Read the model definition and answer for the solid it produces. Units are mm, in the model's axes. Face numbers are marked on the shaded views. A direction names the side the tool comes from. Round coordinates to 2 decimals unless told otherwise and drop trailing zeros. Loops run counter-clockwise (first coordinate to the right, second up) from the corner with the lowest first, then second, coordinate; pieces in that order, holes last. Notation, with made-up numbers: M 3.25,84 L 60.25,84 A31 cw 60.25,111 Z; hole C 52.5,54.25 d5. An arc over 180 degrees is marked long. Write each question's results on one line, items separated by ' | '.
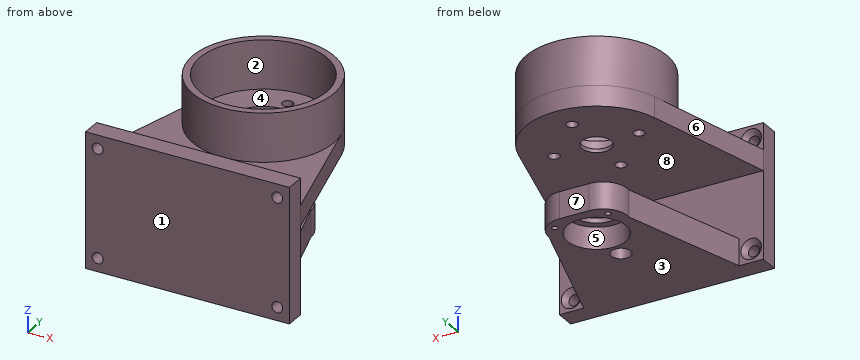
```python
from build123d import *

# Parameters (mm, degrees)
SCHIZZO1_R                   = 12.1
ESTRUSIONE_ESTRUSIONE1_DEPTH = 11
ESTRUSIONE_ESTRUSIONE2_START = -2
SCHIZZO2_R                   = 12.1
SCHIZZO2_R_2                 = 9
ESTRUSIONE_ESTRUSIONE2_DEPTH = 2
SCHIZZO3_R                   = 2.25
TAGLIO_ESTRUSIONE1_DEPTH     = 77.182412669
SMUSSO1_SIZE                 = 2
SCHIZZO4_R                   = 1.25
TAGLIO_ESTRUSIONE2_DEPTH     = 70.679623994
SCHIZZO5_W                   = 84
SCHIZZO5_H                   = 8
ESTRUSIONE_ESTRUSIONE3_DEPTH = 25
SCHIZZO6_R                   = 2.25
SCHIZZO6_R_2                 = 6
ESTRUSIONE_ESTRUSIONE4_DEPTH = 1.5
SCHIZZO7_R                   = 2.25
SCHIZZO7_R_2                 = 13.1
ESTRUSIONE_ESTRUSIONE5_DEPTH = 7
SCHIZZO8_R                   = 29
SCHIZZO8_R_2                 = 26.1
ESTRUSIONE_ESTRUSIONE6_DEPTH = 20
TAGLIO_ESTRUSIONE4_REACH     = 96.311
SCHIZZO9_R                   = 4
SCHIZZO10_W                  = 84
SCHIZZO10_H                  = 8
ESTRUSIONE_ESTRUSIONE7_DEPTH = 11
SCHIZZO11_R                  = 2.25
TAGLIO_ESTRUSIONE5_DEPTH     = 108.816974545
SMUSSO2_SIZE                 = 2


with BuildPart() as part:
    # Schizzo1 → Estrusione-Estrusione1 (new body)
    with BuildSketch(Plane.XY):
        with BuildLine():
            Line((-6.171311325, 16.1), (6.171311325, 16.1))
            ThreePointArc((6.171311325, 16.1), (13.242379137, 13.171067812), (16.171311325, 6.1))
            Line((16.171311325, 6.1), (32, -46.5))
            Line((32, -46.5), (42, -46.5))
            Line((42, -46.5), (42, -54.5))
            Line((42, -54.5), (17, -54.5))
            Line((17, -54.5), (-17, -54.5))
            Line((-17, -54.5), (-42, -54.5))
            Line((-42, -54.5), (-42, -46.5))
            Line((-42, -46.5), (-32, -46.5))
            Line((-32, -46.5), (-16.1, 4.907883736))
            ThreePointArc((-16.1, 4.907883736), (-13.651991863, 12.73622021), (-6.171311325, 16.1))
        make_face()
        Circle(SCHIZZO1_R, mode=Mode.SUBTRACT)
    extrude(amount=ESTRUSIONE_ESTRUSIONE1_DEPTH)

    # Schizzo2 → Estrusione-Estrusione2 (add)
    with BuildSketch(Plane.XY.offset(11).offset(ESTRUSIONE_ESTRUSIONE2_START)):
        Circle(SCHIZZO2_R)
        Circle(SCHIZZO2_R_2, mode=Mode.SUBTRACT)
    extrude(amount=ESTRUSIONE_ESTRUSIONE2_DEPTH)

    # Schizzo3 → Taglio-Estrusione1 (cut, through all)
    with BuildSketch(Plane(origin=(0, -46.5, 0), x_dir=(1, 0, 0), z_dir=(0, 1, 0))):
        with Locations(Location((37, -5.5, 0), (0, 0, 270))):
            Circle(SCHIZZO3_R)
        with Locations(Location((-37, -5.5, 0), (0, 0, 270))):
            Circle(SCHIZZO3_R)
    extrude(amount=-TAGLIO_ESTRUSIONE1_DEPTH, mode=Mode.SUBTRACT)

    # Smusso1
    smusso1_edges = [part.edges().sort_by_distance(p)[0] for p in [
        (37, -46.5, 3.25),
        (-37, -46.5, 3.25),
    ]]
    chamfer(smusso1_edges, length=SMUSSO1_SIZE)

    # Schizzo4 → Taglio-Estrusione2 (cut, through all)
    with BuildSketch(Plane(origin=(0, 0, 0), x_dir=(-1, 0, 0), z_dir=(0, 0, -1))):
        with Locations((-10.910719744, 10.851964601)):
            Circle(SCHIZZO4_R)
        with Locations((10.944459062, 10.817992606)):
            Circle(SCHIZZO4_R)
        with Locations((0, -15.38859776)):
            Circle(SCHIZZO4_R)
    extrude(amount=-TAGLIO_ESTRUSIONE2_DEPTH, mode=Mode.SUBTRACT)

    # Schizzo5 → Estrusione-Estrusione3 (add)
    with BuildSketch(Plane.XY.offset(11)):
        with Locations((0, -50.5)):
            Rectangle(SCHIZZO5_W, SCHIZZO5_H)
    extrude(amount=ESTRUSIONE_ESTRUSIONE3_DEPTH)

    # Schizzo6 → Estrusione-Estrusione4 (add)
    with BuildSketch(Plane.XY.offset(36)):
        with BuildLine():
            Line((-28.073726485, 7.270892739), (-42, -46.5))
            Line((-42, -46.5), (-42, -54.5))
            Line((-42, -54.5), (42, -54.5))
            Line((42, -54.5), (42, -46.5))
            Line((42, -46.5), (28.073726485, 7.270892739))
            ThreePointArc((28.073726485, 7.270892739), (0, 29), (-28.073726485, 7.270892739))
        make_face()
        with Locations((17.5, 0)):
            Circle(SCHIZZO6_R, mode=Mode.SUBTRACT)
        with Locations((0, -17.5)):
            Circle(SCHIZZO6_R, mode=Mode.SUBTRACT)
        with Locations((-17.5, 0)):
            Circle(SCHIZZO6_R, mode=Mode.SUBTRACT)
        with Locations((0, 17.5)):
            Circle(SCHIZZO6_R, mode=Mode.SUBTRACT)
        Circle(SCHIZZO6_R_2, mode=Mode.SUBTRACT)
    extrude(amount=ESTRUSIONE_ESTRUSIONE4_DEPTH)

    # Schizzo7 → Estrusione-Estrusione5 (add)
    with BuildSketch(Plane.XY.offset(37.5)):
        with BuildLine():
            Line((42, -46.5), (28.073726485, 7.270892739))
            ThreePointArc((28.073726485, 7.270892739), (0, 29), (-28.073726485, 7.270892739))
            Line((-28.073726485, 7.270892739), (-42, -46.5))
            Line((-42, -46.5), (-42, -54.5))
            Line((-42, -54.5), (42, -54.5))
            Line((42, -54.5), (42, -46.5))
        make_face()
        with Locations((0, -17.5)):
            Circle(SCHIZZO7_R, mode=Mode.SUBTRACT)
        with Locations((17.5, 0)):
            Circle(SCHIZZO7_R, mode=Mode.SUBTRACT)
        with Locations((0, 17.5)):
            Circle(SCHIZZO7_R, mode=Mode.SUBTRACT)
        with Locations((-17.5, 0)):
            Circle(SCHIZZO7_R, mode=Mode.SUBTRACT)
        Circle(SCHIZZO7_R_2, mode=Mode.SUBTRACT)
    extrude(amount=ESTRUSIONE_ESTRUSIONE5_DEPTH)

    # Schizzo8 → Estrusione-Estrusione6 (add)
    with BuildSketch(Plane.XY.offset(44.5)):
        with Locations(Location((0, 0, 0), (0, 0, 165.479851844))):
            Circle(SCHIZZO8_R)
        Circle(SCHIZZO8_R_2, mode=Mode.SUBTRACT)
    extrude(amount=ESTRUSIONE_ESTRUSIONE6_DEPTH)

    # Schizzo9 → Taglio-Estrusione4 (cut, up to next)
    with BuildSketch(Plane(origin=(0, 0, 0), x_dir=(-1, 0, 0), z_dir=(0, 0, -1)), mode=Mode.PRIVATE) as taglio_estrusione4_sk1:
        with Locations((0, -17.5)):
            Circle(SCHIZZO9_R)
    taglio_estrusione4_tool1 = extrude(taglio_estrusione4_sk1.sketch, amount=-TAGLIO_ESTRUSIONE4_REACH, mode=Mode.PRIVATE) & part.part
    add(taglio_estrusione4_tool1.solids().sort_by_distance((0, -17.5, 0))[0], mode=Mode.SUBTRACT)

    # Schizzo10 → Estrusione-Estrusione7 (add)
    with BuildSketch(Plane.XY.offset(44.5)):
        with Locations((0, -50.5)):
            Rectangle(SCHIZZO10_W, SCHIZZO10_H)
    extrude(amount=ESTRUSIONE_ESTRUSIONE7_DEPTH)

    # Schizzo11 → Taglio-Estrusione5 (cut, through all)
    with BuildSketch(Plane(origin=(0, -46.5, 0), x_dir=(1, 0, 0), z_dir=(0, 1, 0))):
        with Locations(Location((-37, -50, 0), (0, 0, 270))):
            Circle(SCHIZZO11_R)
        with Locations(Location((37, -50, 0), (0, 0, 270))):
            Circle(SCHIZZO11_R)
    extrude(amount=-TAGLIO_ESTRUSIONE5_DEPTH, mode=Mode.SUBTRACT)

    # Smusso2
    smusso2_edges = [part.edges().sort_by_distance(p)[0] for p in [
        (-37, -46.5, 47.75),
        (37, -46.5, 47.75),
    ]]
    chamfer(smusso2_edges, length=SMUSSO2_SIZE)


solid = part.part
```
1. Find section C-C, the plane x = 17.5. Give the vertices of the cut face in (y, z), then the cut area to 3 significant figures.
Completed:
outline: M -54.5,0 L 1.68,0 L 1.68,11 L -46.5,11 L -46.5,36 L -2.25,36 L -2.25,44.5 L -19.36,44.5 L -19.36,64.5 L -23.12,64.5 L -23.12,44.5 L -46.5,44.5 L -46.5,55.5 L -54.5,55.5 Z; M 2.25,36 L 23.12,36 L 23.12,64.5 L 19.36,64.5 L 19.36,44.5 L 2.25,44.5 Z | area: 1,680 mm2
2. Given P1, Ø6, axis at x = -11.5, z = 20.5, coming from the +Y side; P2, Ø22, axis at x = 0, y = 0, coming from the +Z side; P3, Ø5.5, axis at x = 1, z = 4, coming from the +Y side, each flat-ended and moving along its own axis, determine where each tip first touches the part or whether it passes through.
Completed:
P1: stops at y = -46.5 | P2: stops at z = 37.5 | P3: stops at y = 16.1
3. Find section A-A, the plane z = 5.5. Give the vertices of the cut face in (x, y).
Completed:
outline: M -42,-54.5 L -39.25,-54.5 L -39.25,-48.5 L -41.25,-46.5 L -42,-46.5 Z; M -34.75,-54.5 L 34.75,-54.5 L 34.75,-48.5 L 32.75,-46.5 L 32,-46.5 L 16.17,6.1 A10 ccw 6.17,16.1 L -6.17,16.1 A10 ccw -16.1,4.91 L -32,-46.5 L -32.75,-46.5 L -34.75,-48.5 Z; M 39.25,-54.5 L 42,-54.5 L 42,-46.5 L 41.25,-46.5 L 39.25,-48.5 Z; hole C -10.94,10.82 d2.5; hole C 0,0 d24.2; hole C 0,-17.5 d8; hole C 10.91,10.85 d2.5
4. Find section D-D, the plane x = -37. Give the vertices of the cut face in (y, z), then the cut area to 3 significant figures.
Completed:
outline: M -54.5,0 L -46.5,0 L -46.5,1.25 L -48.5,3.25 L -54.5,3.25 Z; M -54.5,7.75 L -48.5,7.75 L -46.5,9.75 L -46.5,36 L -27.19,36 L -27.19,44.5 L -46.5,44.5 L -46.5,45.75 L -48.5,47.75 L -54.5,47.75 Z; M -54.5,52.25 L -48.5,52.25 L -46.5,54.25 L -46.5,55.5 L -54.5,55.5 Z | area: 528 mm2
5. Which of the six approach directions +Z, -Z, +X, -X, +Y, -Y give full straight-line access (tool end or side, diameter ignored) to the marked faces 4, 5, 6, 7 and 8?
Completed:
face 4: +Z | face 5: -Z | face 6: +Z, -Z, -X, +Y | face 7: -Z, +X, -X, +Y | face 8: +X, -X, +Y
6. Find the intervals of material crossed by L1, parallel to X at y = -52.6, z = 5.5; L2, parallel to Y at x = 0, z = 3.25; L3, parallel to Z at x = 5, y = -43, in increasing order.
Completed:
L1: x = -42 to -39.25, -34.75 to 34.75, 39.25 to 42 | L2: y = -54.5 to -21.5, -13.5 to -12.1, 12.1 to 16.1 | L3: z = 0 to 11, 36 to 44.5
7. Determine the mould class of the marked faces 1, 2 and 3 for opening direction Y: released by +Y, released by -Y, zero draft, split by the parting line, or undercut.
Completed:
face 1: released by -Y | face 2: undercut | face 3: zero draft
8. Find section B-B, the plane y = -44. Give the vertices of the cut face in (x, z), then the cut area to 3 significant figures.
Completed:
outline: M -41.35,36 L 41.35,36 L 41.35,44.5 L -41.35,44.5 Z; M -31.23,0 L 31.25,0 L 31.25,11 L -31.23,11 Z | area: 1,390 mm2
